from build123d import *

# Parameters (mm, degrees)
EXTRUDE_1_DEPTH     = 5
SKETCH_3_R          = 5
EXTRUDE_2_DEPTH     = 8
SKETCH_4_R          = 3.5
CUT_EXTRUDE_3_DEPTH = 35.773353009


with BuildPart() as part:
    # 草图1 → 旋转1 (revolve)
    with BuildSketch(Plane(origin=(0, 0, 0), x_dir=(1, 0, 0), z_dir=(0, 1, 0)), mode=Mode.PRIVATE) as revolve_1_sk:
        Polygon((0, 3.047961053), (0, 3.83046551), (4.735897553, 3.83046551), (12, 6.5), (13, 5.5), (15.5, 5.5), (17.339013278, 6.834767245), (20, 6.834767245), (20, 3.417383623), align=None)
    revolve(revolve_1_sk.sketch.rotate(Axis((0, 0, 0), (1, 0, 0)), 180), axis=Axis((0, 0, 0), (1, 0, 0)))

    # 草图2 → 拉伸1 (add)
    with BuildSketch(Plane(origin=(20, 0, 0), x_dir=(0, 0, -1), z_dir=(1, 0, 0))):
        Polygon((8.006144159, -1.111300607), (4.965486636, 6.377873924), (-3.040657522, 7.489174532), (-8.006144159, 1.111300607), (-4.965486636, -6.377873924), (3.040657522, -7.489174532), align=None)
    extrude(amount=EXTRUDE_1_DEPTH)

    # 草图3 → 拉伸2 (add)
    with BuildSketch(Plane(origin=(25, 0, 0), x_dir=(0, 0, -1), z_dir=(1, 0, 0))):
        Circle(SKETCH_3_R)
    extrude(amount=EXTRUDE_2_DEPTH)

    # 草图4 → 拉伸3 (cut, through all)
    with BuildSketch(Plane(origin=(33, 0, 0), x_dir=(0, 0, -1), z_dir=(1, 0, 0))):
        Circle(SKETCH_4_R)
    extrude(amount=-CUT_EXTRUDE_3_DEPTH, mode=Mode.SUBTRACT)


solid = part.part
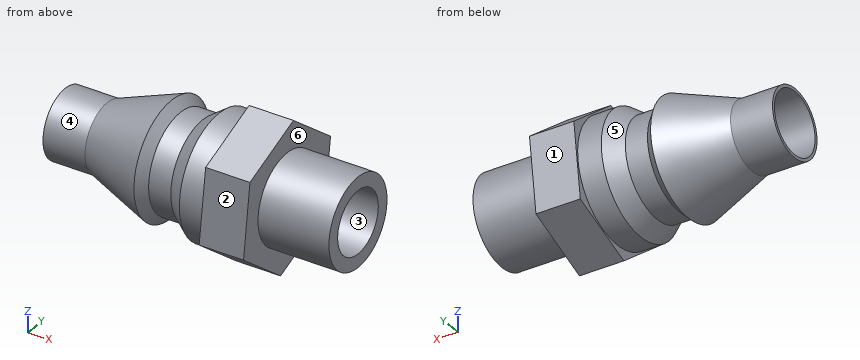
Geometry check sheet. Reference: the model listing, model coordinates, mm. Face numbers are marked on the shaded views. A direction names the side the tool comes from. Round coordinates to 2 decimals unless told otherwise and drop trailing zeros. Loops run counter-clockwise (first coordinate to the right, second up) from the corner with the lowest first, then second, coordinate; pieces in that order, holes last. Notation, with made-up numbers: (-19.75, 0) - (-15.75, 0) arc R37 cw to (-15.75, 38) - close; hole circle Ø11 at (23, 14). An arc over 180 degrees is marked (long way). Answer as CSV lines item,"result".
(1) Release check for a two-part mould opening along Z. For the marked faces 1, 2 and 3 record: released by +Z, released by -Z, zero draft, split by the parting line, or undercut.
Output values:
face 1,"released by -Z"
face 2,"released by +Z"
face 3,"undercut"
(2) Cross-section at C-C, the plane y = 0. Enter the section's corners in (x, z), and give its area (3 significant figures).
Output values:
outline,"(0, -3.83) - (4.74, -3.83) - (12, -6.5) - (13, -5.5) - (15.5, -5.5) - (17.34, -6.83) - (20, -6.83) - (20, -7.55) - (25, -7.55) - (25, -5) - (33, -5) - (33, -3.5) - (0, -3.5) - close; (0, 3.5) - (33, 3.5) - (33, 5) - (25, 5) - (25, 7.55) - (20, 7.55) - (20, 6.83) - (17.34, 6.83) - (15.5, 5.5) - (13, 5.5) - (12, 6.5) - (4.74, 3.83) - (0, 3.83) - close"
area,"134 mm²"
(3) Cross-section at A-A, the plane z = 0. Enter the section's corners in (x, y).
Output values:
outline,"(0, -3.83) - (4.74, -3.83) - (12, -6.5) - (13, -5.5) - (15.5, -5.5) - (17.34, -6.83) - (20, -6.83) - (20, -7.07) - (25, -7.07) - (25, -5) - (33, -5) - (33, -3.5) - (0, -3.5) - close; (0, 3.5) - (33, 3.5) - (33, 5) - (25, 5) - (25, 7.07) - (20, 7.07) - (20, 6.83) - (17.34, 6.83) - (15.5, 5.5) - (13, 5.5) - (12, 6.5) - (4.74, 3.83) - (0, 3.83) - close"
(4) Cross-section at B-B, the plane x = 21.5. Enter the section's corners in (y, z).
Output values:
outline,"(-7.49, -3.04) - (-1.11, -8.01) - (6.38, -4.97) - (7.49, 3.04) - (1.11, 8.01) - (-6.38, 4.97) - close; hole circle Ø7 at (0, 0)"
(5) Cross-section at D-D, the plane x = 18. Enter the section's corners in (y, z).
Output values:
outline,"circle Ø13.67 at (0, 0); hole circle Ø7 at (0, 0)"
(6) Depth check by flat-ended pin: pin 1 Ø8 at (x, y) = (24, -4) entering from +Z; pin 2 Ø8 at (x, z) = (19, 3.5) entering from +Y; pin 3 Ø3 at (x, y) = (16, 4) entering from -Z; pin 4 Ø1.5 at (y, z) = (-1.5, 1.5) entering from -X. Enter the tip coordinate at first touch or a pass-through.
Output values:
pin 1,"stops at z = 7.55"
pin 2,"stops at y = 7.49"
pin 3,"stops at z = -5.98"
pin 4,"passes through"
(7) Set-up check for the marked faces 4, 5 and 6: record each of +Z, -Z, +X, -X, +Y, -Y from which the full face is reachable in a straight line by a thin tool's end or side.
Output values:
face 4,"-X"
face 5,"none"
face 6,"+X"
(8) Material ranges on line 1 along Y through (x, z) = (15, 0); line 2 along Y through (x, z) = (25.5, 0); line 3 along Z through (x, y) = (21, -2), recorded low to high.
Output values:
line 1,"y = -5.5 to -3.5, 3.5 to 5.5"
line 2,"y = -5 to -3.5, 3.5 to 5"
line 3,"z = -7.31 to -2.87, 2.87 to 6.74"
